from build123d import *

# Parameters (mm, degrees)
SKETCH011_R  = 3.2
POCKET_DEPTH = 18.001
CHAMFER_SIZE = 1.5


with BuildPart() as part:
    # Sketch010 → Revolution001 (revolve)
    with BuildSketch(Plane.XZ):
        Polygon((4.2, 20), (4.2, 36), (0, 36), (0, 38), (6.35, 38), (6.35, 20), align=None)
    revolve(axis=Axis((0, 0, 0), (0, 0, 1)))

    # Sketch011 → Pocket (cut, through all)
    with BuildSketch(Plane(origin=(0, 0, 38), x_dir=(-1, 0, 0), z_dir=(0, 0, 1))):
        Circle(SKETCH011_R)
    extrude(amount=-POCKET_DEPTH, mode=Mode.SUBTRACT)

    # Chamfer
    chamfer_edges = [part.edges().sort_by_distance(p)[0] for p in [
        (-6.35, 0, 38),
    ]]
    chamfer(chamfer_edges, length=CHAMFER_SIZE)


solid = part.part
Source: CAD feature listing. Evaluate the final solid. Frame: model axes, mm. A direction names the side the tool comes from. Round coordinates to 2 decimals unless told otherwise and drop trailing zeros. Loops run counter-clockwise (first coordinate to the right, second up) from the corner with the lowest first, then second, coordinate; pieces in that order, holes last. Notation, with made-up numbers: M 38.5,10 L 68.5,10 A24 ccw 68.5,24 Z; hole C -24.75,4 d5. An arc over 180 degrees is marked long. Answer as CSV lines item,"result".
Q1. Line query: line 1 along Y through (x, z) = (0, 27.5); line 2 along X through (y, z) = (-0.5, 22); line 3 along Y through (x, z) = (0, 36.7). Output: solid intervals per line, ascending.
Verdict:
line 1,"y = -6.35 to -4.2, 4.2 to 6.35"
line 2,"x = -6.33 to -4.17, 4.17 to 6.33"
line 3,"y = -6.15 to -3.2, 3.2 to 6.15"
Q2. Reachability of faces 5 (the face through (-3.2, -1, 38)), 6 (the face through (4.006, 1.262, 28.112)) from +Z, -Z, +X, -X, +Y, -Y: full face, straight path, thin tool, end or side. Return the list, or none.
Verdict:
face 5,"+Z, +X, -X, +Y, -Y"
face 6,"-Z"
Q3. Cut plane C-C (z = 31.25). Return the cut outline in (x, y).
Verdict:
outline,"C 0,0 d12.7; hole C 0,0 d8.4"
Q4. Cut plane A-A (y = 0). Return the cut outline in (x, z).
Verdict:
outline,"M -6.35,20 L -4.2,20 L -4.2,36 L -3.2,36 L -3.2,38 L -4.85,38 L -6.35,36.5 Z; M 3.2,36 L 4.2,36 L 4.2,20 L 6.35,20 L 6.35,36.5 L 4.85,38 L 3.2,38 Z"
Q5. Contact query for flat-ended pins moving along their axis: pin 1 (2 mm diameter, centred on x = -4.5, z = 25, fed in from +Y); pin 2 (1.5 mm diameter, centred on y = -2.5, z = 25, fed in from -X); pin 3 (1 mm diameter, centred on x = 2.5, y = 2, fed in from -Z). Output: stop coordinate, or through.
Verdict:
pin 1,"stops at y = 5.3"
pin 2,"stops at x = -6.1"
pin 3,"stops at z = 36"
Q6. Pull-direction query (X, two-part tool) for faces 1 (the face through (-2, -4, 20)), 2 (the face through (2.539, 1.947, 37.014)), 3 (the face through (-3, -2, 36)), 4 (the face through (-1.38, -6.2, 28.13)); classes: +X half, -X half, draft (parallel to the pull), parting line (faces both ways), or undercut.
Verdict:
face 1,"draft"
face 2,"undercut"
face 3,"undercut"
face 4,"parting line"
